Can you work these out from the model? Positions are in its coordinate system, mm. A direction names the side the tool comes from. Coordinates: 2 decimals unless noted, no trailing zeros. Order: outer loops, then holes, each group sorted by start corner. A loop starts at its lowest first (then second) coordinate and runs counter-clockwise, first axis right, second up. Notation, with made-up numbers: (31, 85) -> (70, 85) arc R28 cw to (70, 114) -> close; hole circle Ø8 at (69.5, 36). An arc over 180 degrees is marked (long way). Answer in a Markdown table with one row per item. Add a question column.
1. Imagine slicing it at A-A on y = 0. Write out the boundary of the cut face in (x, z).
2. We'd pull the mould along Y, two halves only. Please class faces 4 (the face through (22.5, 4, -4)), 5 (the face through (11.62, 3.905, -0.867)), 6 (the face through (0.315, 6.835, -1.518)): pulls with the +Y half, pulls with the -Y half, needs draft (parallel to the pull), parting line crosses it, or undercut.
3. Will these pins go through, and if not, where does the flat tip stop? pin 1 (4 mm diameter, centred on x = -0.5, z = 0.5, fed in from +Y); pin 2 (2.5 mm diameter, centred on y = -1, z = 1, fed in from -X); pin 3 (5 mm diameter, centred on x = -9.5, y = 5.5, fed in from +Z); pin 4 (5 mm diameter, centred on y = 0, z = 0, fed in from +X).
4. On a 3-axis mill with a long thin cutter (end or side, diameter ignored), from which of +Z, -Z, +X, -X, +Y, -Y can I reach the whole of each face in a straight line? I mean faces 1 (the face through (-11.88, 3.905, -0.867)), 2 (the face through (-22.5, 4, 4)), 3 (the face through (2.5, 0, 0)). Say none if no direction works.
5. Imagine slicing it at C-C on x = -15. Write out the boundary of the cut face in (y, z), plus the area to 3 significant figures.
6. Imagine slicing it at D-D on z = 6. Write out the boundary of the cut face in (x, y).
7. If I drill on line 1 along Y through (x, z) = (-16.5, 0); line 2 along X through (y, z) = (1.5, -0.75); line 3 along Z through (x, y) = (-12, -2), over which ranges is the centre line in solid material (lowest first)? Write a range as [from, to].
from build123d import *

# Parameters (mm, degrees)
CHAMFER1_SIZE = 1.5


with BuildPart() as part:
    # Sketch1 → Revolve1 (revolve)
    with BuildSketch(Plane.XY, mode=Mode.PRIVATE) as revolve1_sk:
        Polygon((-2.5, 0), (-2.5, 4), (-22.5, 4), (-22.5, 7.00143885), (22.5, 7.00143885), (22.5, 4), (2.5, 4), (2.5, 0), align=None)
    revolve(revolve1_sk.sketch.rotate(Axis((0, 0, 0), (1, 0, 0)), 90), axis=Axis((0, 0, 0), (1, 0, 0)))

    # Chamfer1
    chamfer1_edges = [part.edges().sort_by_distance(p)[0] for p in [
        (22.5, 0, -4),
        (-22.5, 0, -4),
    ]]
    chamfer(chamfer1_edges, length=CHAMFER1_SIZE)


solid = part.part
Answers follow:
| question | item | result |
|---|---|---|
| 1 | outline | (-22.5, -7) -> (22.5, -7) -> (22.5, -5.5) -> (21, -4) -> (2.5, -4) -> (2.5, 4) -> (21, 4) -> (22.5, 5.5) -> (22.5, 7) -> (-22.5, 7) -> (-22.5, 5.5) -> (-21, 4) -> (-2.5, 4) -> (-2.5, -4) -> (-21, -4) -> (-22.5, -5.5) -> close |
| 2 | face 4 | needs draft |
| 2 | face 5 | undercut |
| 2 | face 6 | parting line crosses it |
| 3 | pin 1 | stops at y = 7 |
| 3 | pin 2 | stops at x = -2.5 |
| 3 | pin 3 | stops at z = 6.33 |
| 3 | pin 4 | stops at x = 2.5 |
| 4 | face 1 | -X |
| 4 | face 2 | +Z, -Z, -X, +Y, -Y |
| 4 | face 3 | +X |
| 5 | outline | circle Ø14 at (0, 0); hole circle Ø8 at (0, 0) |
| 5 | area | 104 mm² |
| 6 | outline | (-22.5, -3.61) -> (22.5, -3.61) -> (22.5, 3.61) -> (-22.5, 3.61) -> close |
| 7 | line 1 | y = [-7, -4], [4, 7] |
| 7 | line 2 | x = [-2.5, 2.5] |
| 7 | line 3 | z = [-6.71, -3.46], [3.46, 6.71] |
